Here's how the part is built. I have some questions about the finished solid (model axes, mm). Face numbers are marked on the shaded views. Coordinates: 2 decimals unless noted, no trailing zeros. Write each loop counter-clockwise with the first axis right and the second up, starting at its lowest first coordinate (ties: lowest second). Pieces come first, ordered by that corner, then holes. Notation, with made-up numbers: M 86,69.25 L 101,69.25 A20 ccw 101,103.25 Z; hole C 87,70 d8. An arc over 180 degrees is marked long. Use a Markdown table: item, result.
```python
from build123d import *

# Parameters (mm, degrees)
F0_R     = 120.65
F1_DEPTH = 6.35
F2_R     = 6.35
F3_DEPTH = 38.1
F4_R     = 6.35
F5_DEPTH = 11.3792


with BuildPart() as f1:
    # F0 (on Top) → F1 (new body)
    with BuildSketch(Plane.XY):
        Circle(F0_R)
    extrude(amount=F1_DEPTH)

    # F2 (on face) → F3 (join)
    with BuildSketch(Plane.XY.offset(6.35)):
        with Locations((-93.98, 0)):
            Circle(F2_R)
        with Locations((93.98, 0)):
            Circle(F2_R)
    extrude(amount=F3_DEPTH)

    # F4 (on face) → F5 (join)
    with BuildSketch(Plane.XY.offset(6.35)):
        Polygon((-88.480739, 9.525), (-99.479261, 9.525), (-104.978523, 0), (-99.479261, -9.525), (-88.480739, -9.525), (-82.981477, 0), align=None)
        with Locations((-93.98, 0)):
            Circle(F4_R, mode=Mode.SUBTRACT)
        Polygon((99.479261, 9.525), (88.480739, 9.525), (82.981477, 0), (88.480739, -9.525), (99.479261, -9.525), (104.978523, 0), align=None)
        with Locations((93.98, 0)):
            Circle(F4_R, mode=Mode.SUBTRACT)
    extrude(amount=F5_DEPTH)


solid = f1.part
```
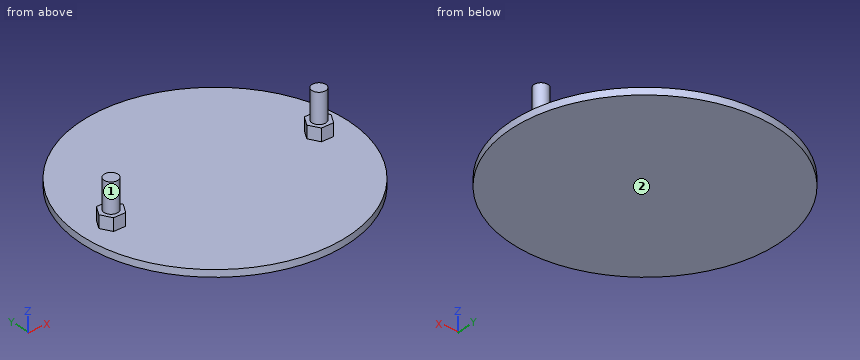
1. Suppose I cut it at D-D on y = -21. Write out the boundary of the cut face in (x, z).
Answers follow:
| item | result |
|---|---|
| outline | M -118.81,0 L 118.81,0 L 118.81,6.35 L -118.81,6.35 Z |
2. Suppose I cut it at C-C on z = 37. Write out the boundary of the cut face in (x, y).
Answers follow:
| item | result |
|---|---|
| outline | C -93.98,0 d12.7; C 93.98,0 d12.7 |
3. I need wall thicknesses on probe 1 along Z at (x, y) = (36, -15); probe 2 along X at (y, z) = (-4, 14); probe 3 along Y at (x, z) = (-93.5, 42). Which ranges of each line are inside material? Lowest first, please.
Answers follow:
| item | result |
|---|---|
| probe 1 | z = 0 to 6.35 |
| probe 2 | x = -102.67 to -85.29, 85.29 to 102.67 |
| probe 3 | y = -6.33 to 6.33 |
4. Suppose I cut it at B-B on x = 0. Write out the boundary of the cut face in (y, z).
Answers follow:
| item | result |
|---|---|
| outline | M -120.65,0 L 120.65,0 L 120.65,6.35 L -120.65,6.35 Z |
5. Suppose I cut it at A-A on z = 12. Write out the boundary of the cut face in (x, y) (3 decimals).
Answers follow:
| item | result |
|---|---|
| outline | M -104.979,0 L -99.479,-9.525 L -88.481,-9.525 L -82.981,0 L -88.481,9.525 L -99.479,9.525 Z; M 82.981,0 L 88.481,-9.525 L 99.479,-9.525 L 104.979,0 L 99.479,9.525 L 88.481,9.525 Z |
6. Will these pins go through, and if not, where does the flat tip stop? pin 1 Ø9 at (x, z) = (-93, 15) entering from -Y (3 decimals); pin 2 Ø5.5 at (x, z) = (-92.5, 9.5) entering from +Y (3 decimals); pin 3 Ø1 at (x, y) = (-36.5, 62) entering from +Z.
Answers follow:
| item | result |
|---|---|
| pin 1 | stops at y = -9.525 |
| pin 2 | stops at y = 9.525 |
| pin 3 | stops at z = 6.35 |
7. We'd pull the mould along X, two halves only. Please class the marked faces 1 and 2: +X half, -X half, draft (parallel to the pull), parting line (faces both ways), or undercut.
Answers follow:
| item | result |
|---|---|
| face 1 | undercut |
| face 2 | draft |
